Source: CAD feature listing. Evaluate the final solid. Frame: model axes, mm. Coordinates: 2 decimals unless noted, no trailing zeros. Write each loop counter-clockwise with the first axis right and the second up, starting at its lowest first coordinate (ties: lowest second). Pieces come first, ordered by that corner, then holes. Notation, with made-up numbers: (50.25, 19) - (89.25, 19) arc R19 ccw to (89.25, 47) - close; hole circle Ø4 at (-31.5, 61.5). An arc over 180 degrees is marked (long way). One line per item, written item: value.
from build123d import *

# Parameters (mm, degrees)
F3_R = 0.275


with BuildPart() as f1:
    # F0 (on Top) → F1 (revolve)
    with BuildSketch(Plane.XY):
        with BuildLine():
            Line((-3.1939512269, 0.7378709646), (-3.25, 0))
            Line((-3.25, 0), (0, 0))
            Line((0, 0), (0, 1.1))
            Line((0, 1.1), (-1.8078035141, 1.1))
            ThreePointArc((-1.8078035141, 1.1), (-1.8195402238, 1.1006911401), (-1.8311146993, 1.1027550071))
            Line((-1.8311146993, 1.1027550071), (-2.2252893382, 1.1972449929))
            ThreePointArc((-2.2252893382, 1.1972449929), (-2.2368638136, 1.1993088599), (-2.2486005233, 1.2))
            Line((-2.2486005233, 1.2), (-2.6953874998, 1.2))
            ThreePointArc((-2.6953874998, 1.2), (-3.0352878658, 1.0666984335), (-3.1939512269, 0.7378709646))
        make_face()
    revolve(axis=Axis((-1.625, 0, 0), (-1, 0, 0)))

    # F2: F1 across face


with BuildPart() as f1_1:
    add(f1.part)
    add(f1.part.mirror(Plane.YZ))



with BuildPart() as f5:
    # F5: sweep along a path in F4
    with BuildLine(Plane.XZ) as f5_path:
        Line((0, 0), (4.28, 0))
        ThreePointArc((4.28, 0), (4.8456854249, -0.2343145751), (5.08, -0.8))
        Line((5.08, -0.8), (5.08, -4.5))
    # F3 (on Right) → F5 (sweep)
    with BuildSketch(Plane.YZ):
        Circle(F3_R)
    sweep(path=f5_path.line)


with BuildPart() as f1_2:
    add(f1_1.part)

    add(f5.part)  # F6 merges F5
    # F6: F5 across plane
    add(f5.part.mirror(Plane.YZ))


solid = f1_2.part
1) Section query A-A on z = -3.6. Output: boundary loops of the cut face in (x, y) (3 decimals).
Values found:
outline: circle Ø0.55 at (-5.08, 0); circle Ø0.55 at (5.08, 0)
2) Section query B-B on x = -1. Output: boundary loops of the cut face in (y, z), then the cut area to 3 significant figures.
Values found:
outline: circle Ø2.2 at (0, 0)
area: 3.80 mm2
3) Contact query for a flat-ended pin moving along its axis: P1, Ø1.5, axis at x = -3.5, z = -1, coming from the +Y side. Output: stop coordinate, or through.
Values found:
P1: y = 1.02
4) Section query C-C on x = -4. Output: boundary loops of the cut face in (y, z) (3 decimals), then the cut area to 3 significant figures.
Values found:
outline: circle Ø0.55 at (0, 0)
area: 0.238 mm2
5) Material intervals for line 1 (Z direction, x = -1, y = 0); line 2 (X direction, y = -0.4, z = 0.8); line 3 (Y direction, x = -0.25, z = -0.85), sorted ascending.
Values found:
line 1: -1.1 to 1.1
line 2: -3.16 to 3.16
line 3: -0.7 to 0.7
